Verification items for the finished model (mm, model axes). Round coordinates to 2 decimals unless told otherwise and drop trailing zeros. Write each loop counter-clockwise with the first axis right and the second up, starting at its lowest first coordinate (ties: lowest second). Pieces come first, ordered by that corner, then holes. Notation, with made-up numbers: M 8.5,81.5 L 27.5,81.5 A18 ccw 27.5,102.5 Z; hole C 18,22 d9. An arc over 180 degrees is marked long. Answer in a Markdown table with one row per item. Add a question column.
1. Sectioned sample at A-A on y = 38.1. Record the cut outline in (x, z).
2. Material ranges on probe 1 along Y at (x, z) = (7, 101.6); probe 2 along Z at (x, y) = (9.5, 26); probe 3 along Y at (x, z) = (8.75, 109), recorded low to high.
3. Draft check along Y on faces 1 (the flat face through (13, 0, 100)), 2 (the cylindrical face through (12.878, 24.152, 104.697)), 3 (the flat face through (13, 39, 0)). Enter one of: pulls with the +Y half, pulls with the -Y half, needs draft (parallel to the pull), parting line crosses it, or undercut.
4. Sectioned sample at B-B on z = 101.6. Record the cut outline in (x, y).
5. Sectioned sample at C-C on x = 17.25. Record the cut outline in (y, z) (1 decimal), plus the area to 3 significant figures.
Autodesk Inventor part; units mm, degrees
ref_plane "YZ Plane" through (0, 0, 0) normal (1, 0, 0) x (0, 1, 0)
ref_plane "XZ Plane" through (0, 0, 0) normal (0, 1, 0) x (-1, 0, 0)
ref_plane "XY Plane" through (0, 0, 0) normal (0, 0, 1) x (1, 0, 0)
sketch "Sketch1" plane through (0, 0, 0) normal (0, 0, 1) x (1, 0, 0)
  line L0 (0, 0) -> (25.4, 0)
  line L1 (25.4, 0) -> (25.4, 76.2)
  line L2 (25.4, 76.2) -> (0, 76.2)
  line L3 (0, 76.2) -> (0, 0)
  dimension "d0" = 25.4
  dimension "d1" = 76.2
extrude "Extrusion1" add sketch "Sketch1" along normal blind 203.2
sketch "Sketch2" plane through (25.4, 0, 0) normal (1, 0, 0) x (0, 0, -1)
  circle A0 centre (-101.6, 38.1) radius 14.2875
  point P0 (0, 0)
  dimension "d4" = 28.575
extrude "Extrusion2" cut sketch "Sketch2" against normal up to next
properties part number "mountingBoard"
Geometry check:
| question | item | result |
|---|---|---|
| 1 | outline | M 0,0 L 25.4,0 L 25.4,87.31 L 0,87.31 Z; M 0,115.89 L 25.4,115.89 L 25.4,203.2 L 0,203.2 Z |
| 2 | probe 1 | y = 0 to 23.81, 52.39 to 76.2 |
| 2 | probe 2 | z = 0 to 94, 109.2 to 203.2 |
| 2 | probe 3 | y = 0 to 25.88, 50.32 to 76.2 |
| 3 | face 1 | pulls with the -Y half |
| 3 | face 2 | undercut |
| 3 | face 3 | needs draft |
| 4 | outline | M 0,0 L 25.4,0 L 25.4,23.81 L 0,23.81 Z; M 0,52.39 L 25.4,52.39 L 25.4,76.2 L 0,76.2 Z |
| 5 | outline | M 0,0 L 76.2,0 L 76.2,203.2 L 0,203.2 Z; hole C 38.1,101.6 d28.6 |
| 5 | area | 14,800 mm2 |
